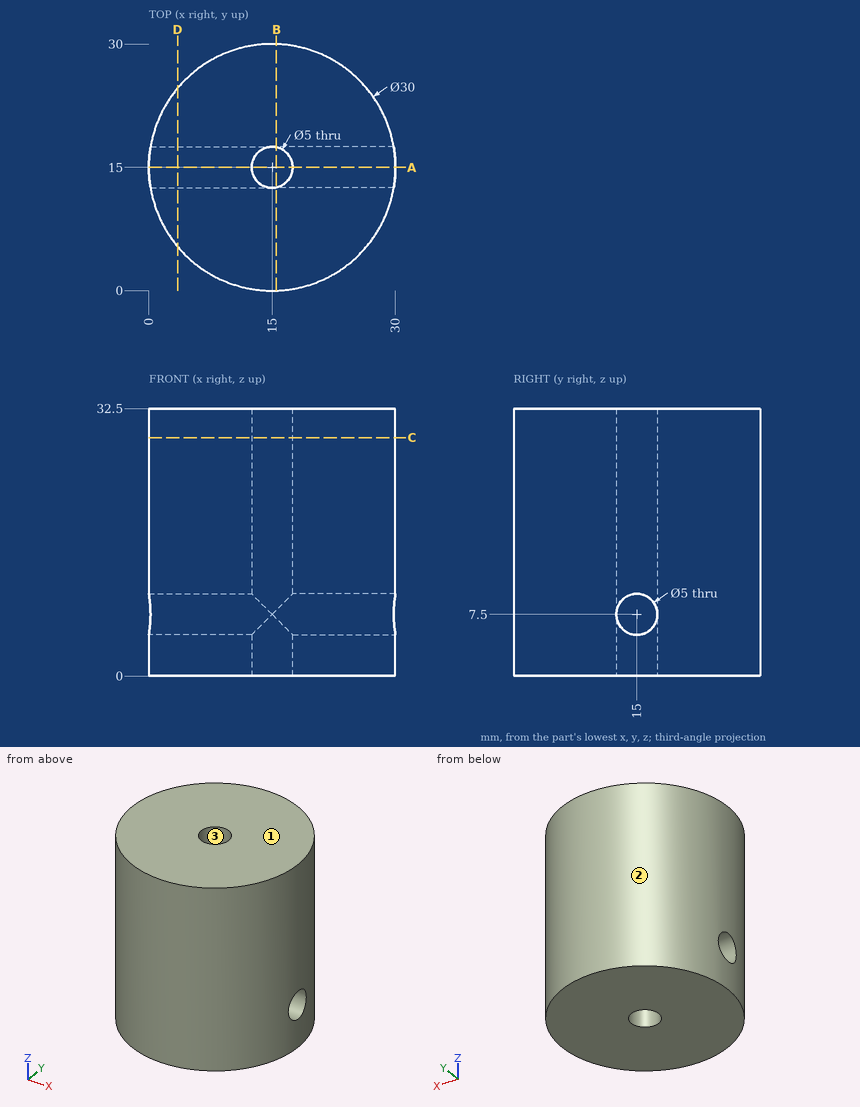
Could you check a few things on this drawing? It's one solid part, dimensions in mm from its lowest x, y, z. Give positions to 0.01 mm unless a question says otherwise; leave off trailing zeros. Order: outer loops, then holes, each group sorted by start corner. A loop starts at its lowest first (then second) coordinate and runs counter-clockwise, first axis right, second up. Notation, with made-up numbers: (30.5, 39.25) - (38.5, 39.25) arc R18 ccw to (38.5, 61.25) - close; hole circle Ø1 at (68.25, -11). An arc over 180 degrees is marked (long way). Return JSON: item names as keys, results as strings. Group by question number.
Q1. Suppose I cut it at D-D, the plane x = 3.5. Please give me the cut outline in (y, z).
Q2. Please list where these lines run through material, in increasing order: line 1 along Y through (x, z) = (15, 2); line 2 along X through (y, z) = (16.5, 4.5); line 3 along X through (y, z) = (14, 26.5). Write a range as [from, to].
Q3. Will these pins go through, and if not, where does the flat tip stop? pin 1 Ø10 at (x, z) = (9, 16.5) entering from -Y; pin 2 Ø8 at (y, z) = (9, 5.5) entering from +X; pin 3 Ø2 at (y, z) = (10.5, 24.5) entering from -X.
Q4. Thinking about a two-plate mould opening in X: for the marked faces 1, 2 and 3, which applies, pulls with the +X half, pulls with the -X half, needs draft (parallel to the pull), parting line crosses it, or undercut?
Q5. Suppose I cut it at B-B, the plane x = 15.5. Please give me the cut outline in (y, z).
Q6. Suppose I cut it at A-A, the plane y = 15. Please give me the cut outline in (x, z), and give its area (4 significant figures).
Q7. Suppose I cut it at C-C, the plane z = 29. Please give me the cut outline in (x, y).
Resolved:
{
 "1": {"outline": "(5.37, 0) - (24.63, 0) - (24.63, 32.5) - (5.37, 32.5) - close; hole circle Ø5 at (15, 7.5)"},
 "2": {"line 1": "y = [0, 12.5], [17.5, 30]", "line 2": "x = [0.08, 13], [17, 29.92]", "line 3": "x = [0.03, 12.71], [17.29, 29.97]"},
 "3": {"pin 1": "stops at y = 0.03", "pin 2": "stops at x = 29.87", "pin 3": "stops at x = 0.41"},
 "4": {"face 1": "needs draft", "face 2": "parting line crosses it", "face 3": "undercut"},
 "5": {"outline": "(0.01, 0) - (12.55, 0) - (12.55, 7) arc R2.5 cw to (12.55, 8) - (12.55, 32.5) - (0.01, 32.5) - close; (17.45, 0) - (29.99, 0) - (29.99, 32.5) - (17.45, 32.5) - (17.45, 8) arc R2.5 cw to (17.45, 7) - close"},
 "6": {"outline": "(0, 0) - (12.5, 0) - (12.5, 5) - (0, 5) - close; (0, 10) - (12.5, 10) - (12.5, 32.5) - (0, 32.5) - close; (17.5, 0) - (30, 0) - (30, 5) - (17.5, 5) - close; (17.5, 10) - (30, 10) - (30, 32.5) - (17.5, 32.5) - close", "area": "687.5 mm2"},
 "7": {"outline": "circle Ø30 at (15, 15); hole circle Ø5 at (15, 15)"}
}
